Can you work these out from the drawing? Everything is in mm from the part's minimum corner. A direction names the side the tool comes from. Coordinates: 2 decimals unless noted, no trailing zeros. Order: outer loops, then holes, each group sorted by start corner. A loop starts at its lowest first (then second) coordinate and runs counter-clockwise, first axis right, second up. Notation, with made-up numbers: (23, 56.5) -> (36, 56.5) arc R10 cw to (36, 70.5) -> close; hole circle Ø7 at (34, -25). An arc over 180 degrees is marked (long way). Use a Markdown table: item, result. Add a question column.
1) If I drill on L1, parallel to Z at x = 22.5, y = 2.1; L2, parallel to Y at x = 11, z = 37; L3, parallel to Z at x = 39, y = 2.45, over which ranges is the centre line in solid material (lowest first)? Write a range as [from, to].
2) If we section it at C-C (z = 39): Write out the boundary of the cut face in (x, y).
3) If we section it at B-B (z = 22.5): Write out the boundary of the cut face in (x, y).
4) If we section it at D-D (y = 8): Write out the boundary of the cut face in (x, z).
5) Will these pins go through, and if not, where does the flat tip stop? pin 1 Ø5 at (x, z) = (11, 15) entering from -Y; pin 2 Ø4 at (x, y) = (29, 4.5) entering from -Z; pin 3 Ø1.5 at (y, z) = (6, 21.5) entering from -X; pin 4 Ø4 at (x, z) = (39, 22.5) entering from +Y.
6) Which directions (+Z, -Z, +X, -X, +Y, -Y) give clear straight access to the entire face, cutting with the end or side of a thin tool? Please do the marked faces 1, 2 and 3.
7) If we section it at A-A (x = 22.5): Write out the boundary of the cut face in (y, z), plus the area to 3 significant figures.
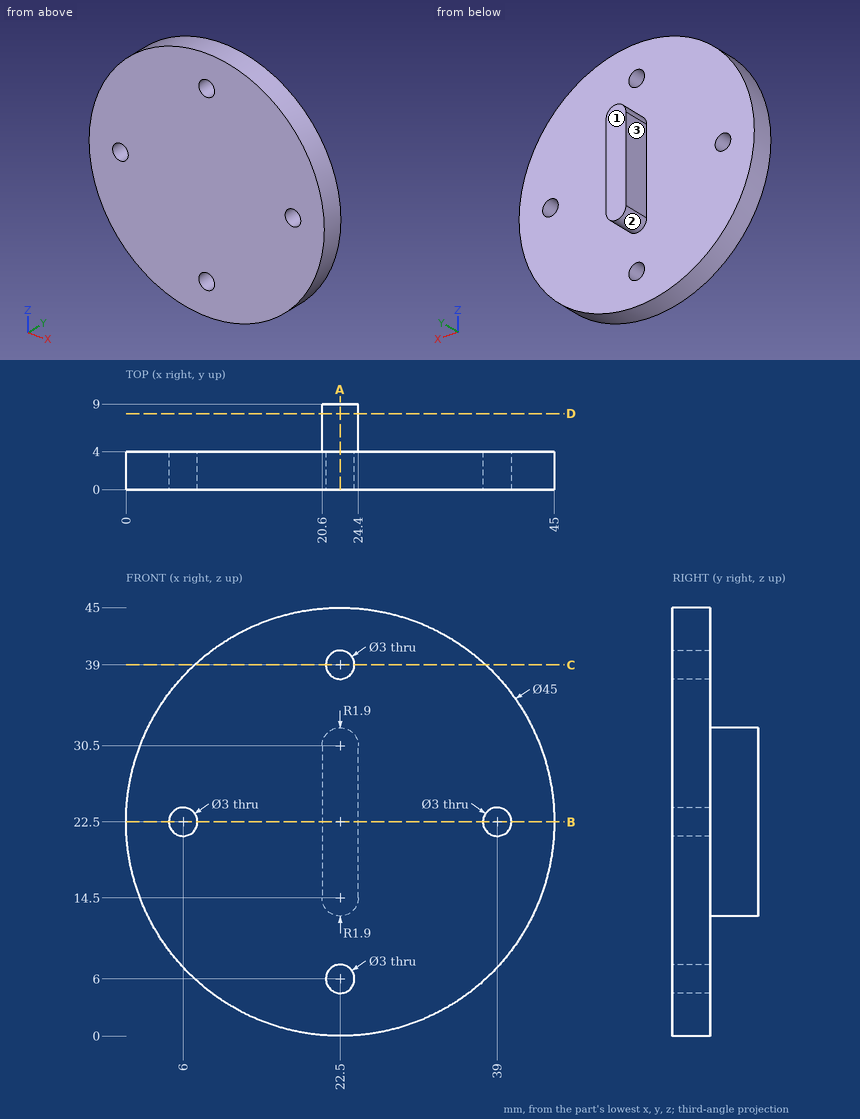
Answer sheet:
| question | item | result |
|---|---|---|
| 1 | L1 | [0, 4.5], [7.5, 37.5], [40.5, 45] |
| 1 | L2 | [0, 4] |
| 1 | L3 | [7.2, 21], [24, 37.8] |
| 2 | outline | (7.2, 0) -> (21, 0) -> (21, 4) -> (7.2, 4) -> close; (24, 0) -> (37.8, 0) -> (37.8, 4) -> (24, 4) -> close |
| 3 | outline | (0, 0) -> (4.5, 0) -> (4.5, 4) -> (0, 4) -> close; (7.5, 0) -> (37.5, 0) -> (37.5, 4) -> (24.4, 4) -> (24.4, 9) -> (20.6, 9) -> (20.6, 4) -> (7.5, 4) -> close; (40.5, 0) -> (45, 0) -> (45, 4) -> (40.5, 4) -> close |
| 4 | outline | (20.6, 14.5) arc R1.9 ccw to (24.4, 14.5) -> (24.4, 30.5) arc R1.9 ccw to (20.6, 30.5) -> close |
| 5 | pin 1 | y = 0 |
| 5 | pin 2 | z = 0.47 |
| 5 | pin 3 | x = 20.6 |
| 5 | pin 4 | y = 4 |
| 6 | face 1 | +Z, -Z, +X, -X, +Y |
| 6 | face 2 | -Z, +Y |
| 6 | face 3 | +Z, -Z, -X, +Y |
| 7 | outline | (0, 0) -> (4, 0) -> (4, 4.5) -> (0, 4.5) -> close; (0, 7.5) -> (4, 7.5) -> (4, 12.6) -> (9, 12.6) -> (9, 32.4) -> (4, 32.4) -> (4, 37.5) -> (0, 37.5) -> close; (0, 40.5) -> (4, 40.5) -> (4, 45) -> (0, 45) -> close |
| 7 | area | 255 mm2 |
